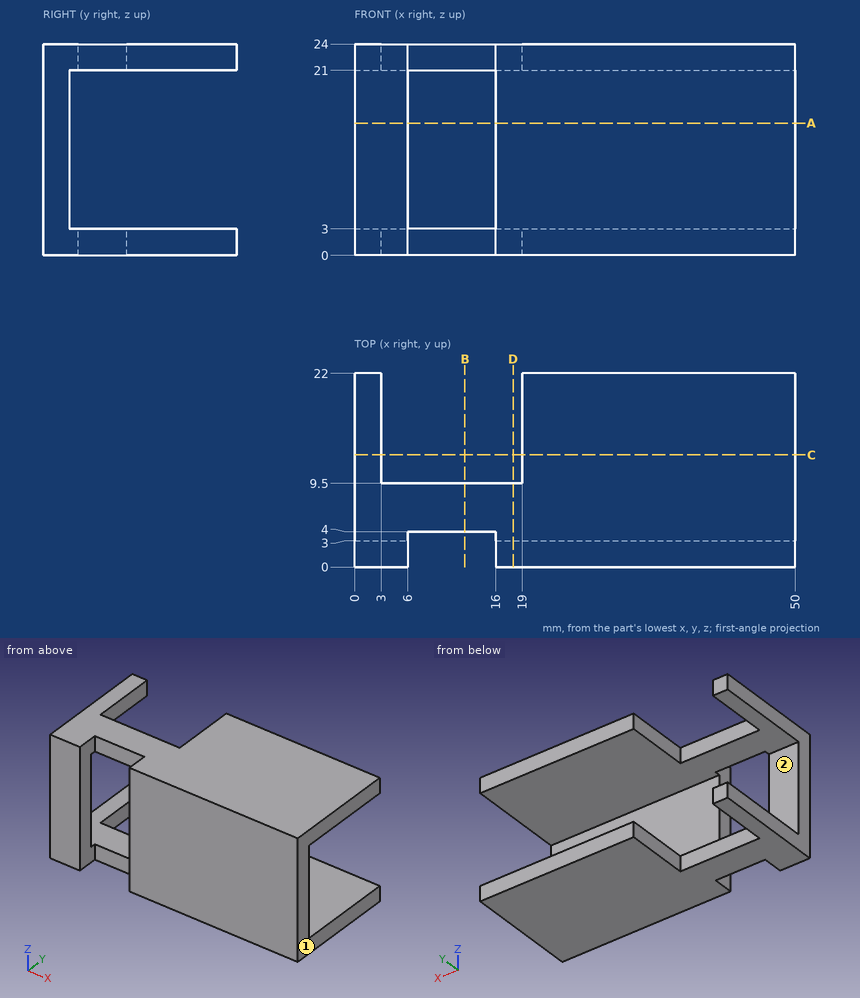
For this review, use the dimensioned drawing (mm, ordinates from the lowest corner) and the shaded views. A direction names the side the tool comes from. Give positions to 0.01 mm unless a question says otherwise; leave off trailing zeros. Loops run counter-clockwise (first coordinate to the right, second up) from the corner with the lowest first, then second, coordinate; pieces in that order, holes last.
Item 1: Take a section at A-A, the plane z = 15. State the section outline as (x, y) points.
Item 2: Take a section at C-C, the plane y = 12.75. State the section outline as (x, z) points.
Item 3: Take a section at D-D, the plane x = 18. State the section outline as (y, z) points.
Item 4: Tool access review of the marked faces 1 and 2: name each direction out of +Z, -Z, +X, -X, +Y, -Y from which nothing blocks a thin tool from reaching the whole face with its end or side.
Item 5: Take a section at B-B, the plane x = 12.5. State the section outline as (y, z) points, and give its area (3 significant figures).
Item 6: For line 1 along Z through (x, y) = (46, 17.5); line 2 along Y through (x, z) = (46.5, 9.75); line 3 along X through (y, z) = (2.5, 7.75), list the stretches that pass through material, from the lowest coordinate up.
Item 7: Insertion check: pin 1 (2 mm diameter, centred on x = 26.5, z = 17.5, fed in from +Y); pin 2 (0.9 mm diameter, centred on x = 13, z = 22, fed in from +Y); pin 3 (3.5 mm diameter, centred on x = 11, z = 22, fed in from -Y). Each pin has a flat end and moves straight along its axis. Give the tip position at first contact, or say it passes through.
Calculated:
1. outline: (0, 0) - (6, 0) - (6, 3) - (0, 3) - close; (16, 0) - (50, 0) - (50, 3) - (16, 3) - close
2. outline: (0, 0) - (3, 0) - (3, 3) - (0, 3) - close; (0, 21) - (3, 21) - (3, 24) - (0, 24) - close; (19, 0) - (50, 0) - (50, 3) - (19, 3) - close; (19, 21) - (50, 21) - (50, 24) - (19, 24) - close
3. outline: (0, 0) - (9.5, 0) - (9.5, 3) - (3, 3) - (3, 21) - (9.5, 21) - (9.5, 24) - (0, 24) - close
4. face 1: +Z, -Z, +X, +Y, -Y
4. face 2: +X, -X, +Y
5. outline: (4, 0) - (9.5, 0) - (9.5, 3) - (4, 3) - close; (4, 21) - (9.5, 21) - (9.5, 24) - (4, 24) - close
5. area: 33.0 mm2
6. line 1: z = 0 to 3, 21 to 24
6. line 2: y = 0 to 3
6. line 3: x = 0 to 6, 16 to 50
7. pin 1: stops at y = 3
7. pin 2: stops at y = 9.5
7. pin 3: stops at y = 4
